Here's how the part is built. I have some questions about the finished solid (model axes, mm). A direction names the side the tool comes from. Coordinates: 2 decimals unless noted, no trailing zeros. Write each loop counter-clockwise with the first axis right and the second up, starting at its lowest first coordinate (ties: lowest second). Pieces come first, ordered by that corner, then holes. Notation, with made-up numbers: M 82,42.25 L 124,42.25 A24 ccw 124,81.25 Z; hole C -4.75,39.5 d3. An arc over 180 degrees is marked long. Use a Markdown table: item, result.
```python
from build123d import *

# Parameters (mm, degrees)
F3_DEPTH = 50
F5_DEPTH = 50


with BuildPart() as f1:
    # F0 (on Front) → F1 (revolve)
    with BuildSketch(Plane.XZ):
        Polygon((39, 30), (0, 30), (0, 0), (39, 0), (39, 16.5), (34, 16.5), (34, 20), (39, 20), (39, 22.5), (34, 22.5), (34, 24.5), (39, 24.5), (39, 27), (34, 27), (34, 28), (39, 28), align=None)
    revolve(axis=Axis((0, 0, 15), (0, 0, -1)))

    # F2 (on Right) → F3 (cut, symmetric)
    with BuildSketch(Plane.YZ):
        with BuildLine():
            Line((-36.911555, 0), (-2.806354, 0))
            ThreePointArc((-2.806354, 0), (-8.50987, 1.785993), (-12.176097, 6.506018))
            Line((-12.176097, 6.506018), (-12.91741, 8.493982))
            ThreePointArc((-12.91741, 8.493982), (-16.583638, 13.214007), (-22.287154, 15))
            Line((-22.287154, 15), (-36.911555, 15))
            Line((-36.911555, 15), (-36.911555, 0))
        make_face()
        with BuildLine():
            Line((36.911555, 15), (22.287154, 15))
            ThreePointArc((22.287154, 15), (16.583638, 13.214007), (12.91741, 8.493982))
            Line((12.91741, 8.493982), (12.176097, 6.506018))
            ThreePointArc((12.176097, 6.506018), (8.50987, 1.785993), (2.806354, 0))
            Line((2.806354, 0), (36.911555, 0))
            Line((36.911555, 0), (36.911555, 15))
        make_face()
    extrude(amount=F3_DEPTH, both=True, mode=Mode.SUBTRACT)

    # F4 (on Right) → F5 (cut, symmetric)
    with BuildSketch(Plane.YZ):
        with BuildLine():
            ThreePointArc((0, 15.75), (-7.5, 8.25), (0, 0.75))
            Line((0, 0.75), (0, 8.25))
            Line((0, 8.25), (0, 15.75))
        make_face()
        with BuildLine():
            Line((0, 8.25), (0, 0.75))
            ThreePointArc((0, 0.75), (5.303301, 2.946699), (7.5, 8.25))
            ThreePointArc((7.5, 8.25), (5.303301, 13.553301), (0, 15.75))
            Line((0, 15.75), (0, 8.25))
        make_face()
    extrude(amount=F5_DEPTH, both=True, mode=Mode.SUBTRACT)


solid = f1.part
```
1. We'd pull the mould along Y, two halves only. Please class faces 4 (the face through (-0.54, -8.44, 1.74)), 5 (the face through (-5.077, -38.668, 25.768)), 6 (the face through (1, 0, 0)): +Y half, -Y half, draft (parallel to the pull), parting line (faces both ways), or undercut.
Answers follow:
| item | result |
|---|---|
| face 4 | undercut |
| face 5 | parting line |
| face 6 | draft |
2. Suppose I cut it at B-B on y = -24.5. Write out the boundary of the cut face in (x, z).
Answers follow:
| item | result |
|---|---|
| outline | M -30.34,15 L 30.34,15 L 30.34,16.5 L 23.57,16.5 L 23.57,20 L 30.34,20 L 30.34,22.5 L 23.57,22.5 L 23.57,24.5 L 30.34,24.5 L 30.34,27 L 23.57,27 L 23.57,28 L 30.34,28 L 30.34,30 L -30.34,30 L -30.34,28 L -23.57,28 L -23.57,27 L -30.34,27 L -30.34,24.5 L -23.57,24.5 L -23.57,22.5 L -30.34,22.5 L -30.34,20 L -23.57,20 L -23.57,16.5 L -30.34,16.5 Z |
3. Suppose I cut it at D-D on y = -16.5. Write out the boundary of the cut face in (x, z), and give its area (3 significant figures).
Answers follow:
| item | result |
|---|---|
| outline | M -35.34,13.16 L 35.34,13.16 L 35.34,16.5 L 29.73,16.5 L 29.73,20 L 35.34,20 L 35.34,22.5 L 29.73,22.5 L 29.73,24.5 L 35.34,24.5 L 35.34,27 L 29.73,27 L 29.73,28 L 35.34,28 L 35.34,30 L -35.34,30 L -35.34,28 L -29.73,28 L -29.73,27 L -35.34,27 L -35.34,24.5 L -29.73,24.5 L -29.73,22.5 L -35.34,22.5 L -35.34,20 L -29.73,20 L -29.73,16.5 L -35.34,16.5 Z |
| area | 1,120 mm2 |
4. Suppose I cut it at C-C on z = 26. Write out the boundary of the cut face in (x, y), and give its area (3 significant figures).
Answers follow:
| item | result |
|---|---|
| outline | C 0,0 d78 |
| area | 4,780 mm2 |
5. I need wall thicknesses on probe 1 along Z at (x, y) = (-22.5, 27); probe 2 along Y at (x, z) = (-6, 11); probe 3 along Y at (x, z) = (2.5, 14). Which ranges of each line are inside material? Lowest first, please.
Answers follow:
| item | result |
|---|---|
| probe 1 | z = 15 to 16.5, 20 to 22.5, 24.5 to 27, 28 to 30 |
| probe 2 | y = -38.54 to -36.91, -14.29 to -6.98, 6.98 to 14.29, 36.91 to 38.54 |
| probe 3 | y = -38.92 to -36.91, -17.93 to -4.82, 4.82 to 17.93, 36.91 to 38.92 |
6. Will these pins go through, and if not, where does the flat tip stop? pin 1 Ø5 at (x, z) = (15, 23.5) entering from -Y; pin 2 Ø6 at (x, z) = (4, 18) entering from +Y; pin 3 Ø4 at (y, z) = (29, 15.5) entering from +X.
Answers follow:
| item | result |
|---|---|
| pin 1 | stops at y = -36.87 |
| pin 2 | stops at y = 38.97 |
| pin 3 | stops at x = 28.14 |
7. Suppose I cut it at A-A on z = 2.5. Write out the boundary of the cut face in (x, y), and give its area (3 significant figures).
Answers follow:
| item | result |
|---|---|
| outline | M -38.7,-4.82 A39 ccw -37.85,-9.42 L 37.85,-9.42 A39 ccw 38.7,-4.82 Z; M -38.7,4.82 L 38.7,4.82 A39 ccw 37.85,9.42 L -37.85,9.42 A39 ccw Z; M -12.59,-36.91 A39 ccw 12.59,-36.91 Z; M -12.59,36.91 L 12.59,36.91 A39 ccw Z |
| area | 776 mm2 |
8. Which directions (+Z, -Z, +X, -X, +Y, -Y) give clear straight access to the entire face, cutting with the end or side of a thin tool? Please do faces 1 (the face through (37.2, -11.71, 10.2)), 2 (the face through (12, -32, 20)), 3 (the face through (-0.519, -12.542, 7.486)).
Answers follow:
| item | result |
|---|---|
| face 1 | +Z, -Z |
| face 2 | none |
| face 3 | -Z, +X, -X |
